```python
from build123d import *

# Parameters (mm, degrees)
SKETCH1_W                                           = 45
SKETCH1_H                                           = 40
BOSS_EXTRUDE1_DEPTH                                 = 29
SKETCH33_W                                          = 34
SKETCH33_H                                          = 35
CUT_EXTRUDE7_DEPTH                                  = 67.828137786
SKETCH39_W                                          = 45
SKETCH39_H                                          = 9
BOSS_EXTRUDE2_DEPTH                                 = 3
CUT_EXTRUDE6_DEPTH                                  = 69.6658576
CUT_EXTRUDE6_DEPTH_BACK                             = 69.6658576
SKETCH21_R                                          = 1.75
SKETCH34_R                                          = 3
CUT_EXTRUDE8_DEPTH                                  = 23
CBORE_FOR_M3_HEX_SOCKET_HEAD_CAP_SCREW1_D           = 3.4
CBORE_FOR_M3_HEX_SOCKET_HEAD_CAP_SCREW1_CBORE_D     = 6.5
CBORE_FOR_M3_HEX_SOCKET_HEAD_CAP_SCREW1_CBORE_DEPTH = 3.4
CBORE_FOR_M3_HEX_SOCKET_HEAD_CAP_SCREW2_D           = 3.4
CBORE_FOR_M3_HEX_SOCKET_HEAD_CAP_SCREW2_CBORE_D     = 6.5
CBORE_FOR_M3_HEX_SOCKET_HEAD_CAP_SCREW2_CBORE_DEPTH = 3.4
FILLET1_R                                           = 4.5
SKETCH40_W                                          = 43
SKETCH40_H                                          = 2
CUT_EXTRUDE9_DEPTH                                  = 69.665857708


with BuildPart() as part:
    # Sketch1 → Boss-Extrude1 (new body)
    with BuildSketch(Plane(origin=(0, 0, 0), x_dir=(1, 0, 0), z_dir=(0, 1, 0))):
        with Locations((22.5, 20)):
            Rectangle(SKETCH1_W, SKETCH1_H)
    extrude(amount=BOSS_EXTRUDE1_DEPTH)

    # Sketch33 → Cut-Extrude7 (cut, through all)
    with BuildSketch(Plane(origin=(0, 29, 0), x_dir=(1, 0, 0), z_dir=(0, 1, 0))):
        with Locations((28, 17.5)):
            Rectangle(SKETCH33_W, SKETCH33_H)
    extrude(amount=-CUT_EXTRUDE7_DEPTH, mode=Mode.SUBTRACT)

    # Sketch39 → Boss-Extrude2 (add)
    with BuildSketch(Plane(origin=(0, 0, -40), x_dir=(-1, 0, 0), z_dir=(0, 0, -1))):
        with Locations((-22.5, 4.5)):
            Rectangle(SKETCH39_W, SKETCH39_H)
    extrude(amount=BOSS_EXTRUDE2_DEPTH)

    # Sketch21 → Cut-Extrude6 (cut, two sides: drawn at the far end of the back side and taken through both)
    with BuildSketch(Plane(origin=(0, 29, 0), x_dir=(1, 0, 0), z_dir=(0, 1, 0)).offset(-CUT_EXTRUDE6_DEPTH_BACK)):
        with Locations(Location((6.5, 39.5, 0), (0, 0, 270))):
            Circle(SKETCH21_R)
        with Locations(Location((6.5, 8.5, 0), (0, 0, 270))):
            Circle(SKETCH21_R)
        with Locations(Location((37.5, 39.5, 0), (0, 0, 270))):
            Circle(SKETCH21_R)
    extrude(amount=CUT_EXTRUDE6_DEPTH + CUT_EXTRUDE6_DEPTH_BACK, mode=Mode.SUBTRACT)

    # Sketch34 → Cut-Extrude8 (cut)
    with BuildSketch(Plane(origin=(0, 29, 0), x_dir=(1, 0, 0), z_dir=(0, 1, 0))):
        with Locations(Location((6.5, 8.5, 0), (0, 0, 270))):
            Circle(SKETCH34_R)
        with Locations(Location((6.5, 39.5, 0), (0, 0, 270))):
            Circle(SKETCH34_R)
        with Locations(Location((37.5, 39.5, 0), (0, 0, 270))):
            Circle(SKETCH34_R)
    extrude(amount=-CUT_EXTRUDE8_DEPTH, mode=Mode.SUBTRACT)

    # CBORE for M3 Hex Socket Head Cap Screw1 (through all)
    with Locations(Plane(origin=(11, 0, 0), x_dir=(0, 0, -1), z_dir=(1, 0, 0))):
        with Locations((16, 19), (30, 19)):
            CounterBoreHole(CBORE_FOR_M3_HEX_SOCKET_HEAD_CAP_SCREW1_D / 2, CBORE_FOR_M3_HEX_SOCKET_HEAD_CAP_SCREW1_CBORE_D / 2, CBORE_FOR_M3_HEX_SOCKET_HEAD_CAP_SCREW1_CBORE_DEPTH)

    # CBORE for M3 Hex Socket Head Cap Screw2 (through all)
    with Locations(Plane.XY.offset(-35)):
        with Locations((16, 19), (30, 19)):
            CounterBoreHole(CBORE_FOR_M3_HEX_SOCKET_HEAD_CAP_SCREW2_D / 2, CBORE_FOR_M3_HEX_SOCKET_HEAD_CAP_SCREW2_CBORE_D / 2, CBORE_FOR_M3_HEX_SOCKET_HEAD_CAP_SCREW2_CBORE_DEPTH)

    # Fillet1
    # the kernel refuses this fillet: 4.5 mm, written as the material it takes off along each edge
    with BuildSketch(Plane(origin=(45, 29, -35), x_dir=(0, 0, -1), z_dir=(0, -1, 0))) as fillet1_piece_1:
        with BuildLine():
            CenterArc((FILLET1_R, -FILLET1_R), FILLET1_R, 90, 90)
            Line((0, -FILLET1_R), (-FILLET1_R * 0.02, -FILLET1_R))
            Line((-FILLET1_R * 0.02, -FILLET1_R), (-FILLET1_R * 0.02, FILLET1_R * 0.02))
            Line((-FILLET1_R * 0.02, FILLET1_R * 0.02), (FILLET1_R, FILLET1_R * 0.02))
            Line((FILLET1_R, FILLET1_R * 0.02), (FILLET1_R, 0))
        make_face()
    extrude(amount=29, mode=Mode.SUBTRACT)
    with BuildSketch(Plane(origin=(11, 29, 0), x_dir=(-1, 0, 0), z_dir=(0, -1, 0))) as fillet1_piece_2:
        with BuildLine():
            CenterArc((FILLET1_R, FILLET1_R), FILLET1_R, 180, 90)
            Line((0, FILLET1_R), (-FILLET1_R * 0.02, FILLET1_R))
            Line((-FILLET1_R * 0.02, FILLET1_R), (-FILLET1_R * 0.02, -FILLET1_R * 0.02))
            Line((-FILLET1_R * 0.02, -FILLET1_R * 0.02), (FILLET1_R, -FILLET1_R * 0.02))
            Line((FILLET1_R, -FILLET1_R * 0.02), (FILLET1_R, 0))
        make_face()
    extrude(amount=29, mode=Mode.SUBTRACT)
    with BuildSketch(Plane(origin=(11, 29, -35), x_dir=(0, 0, -1), z_dir=(1, 0, 0))) as fillet1_piece_3:
        with BuildLine():
            CenterArc((FILLET1_R, -FILLET1_R), FILLET1_R, 90, 90)
            Line((0, -FILLET1_R), (-FILLET1_R * 0.02, -FILLET1_R))
            Line((-FILLET1_R * 0.02, -FILLET1_R), (-FILLET1_R * 0.02, FILLET1_R * 0.02))
            Line((-FILLET1_R * 0.02, FILLET1_R * 0.02), (FILLET1_R, FILLET1_R * 0.02))
            Line((FILLET1_R, FILLET1_R * 0.02), (FILLET1_R, 0))
        make_face()
    extrude(amount=34, mode=Mode.SUBTRACT)
    with BuildSketch(Plane(origin=(11, 29, 0), x_dir=(0, -1, 0), z_dir=(0, 0, -1))) as fillet1_piece_4:
        with BuildLine():
            CenterArc((FILLET1_R, FILLET1_R), FILLET1_R, 180, 90)
            Line((0, FILLET1_R), (-FILLET1_R * 0.02, FILLET1_R))
            Line((-FILLET1_R * 0.02, FILLET1_R), (-FILLET1_R * 0.02, -FILLET1_R * 0.02))
            Line((-FILLET1_R * 0.02, -FILLET1_R * 0.02), (FILLET1_R, -FILLET1_R * 0.02))
            Line((FILLET1_R, -FILLET1_R * 0.02), (FILLET1_R, 0))
        make_face()
    extrude(amount=35, mode=Mode.SUBTRACT)
    with BuildSketch(Plane(origin=(11, 29, -35), x_dir=(0, 0, -1), z_dir=(1, 0, 0))) as fillet1_piece_5a_section:
        with BuildLine():
            CenterArc((FILLET1_R, -FILLET1_R), FILLET1_R, 90, 90)
            Line((0, -FILLET1_R), (-FILLET1_R * 0.02, -FILLET1_R))
            Line((-FILLET1_R * 0.02, -FILLET1_R), (-FILLET1_R * 0.02, FILLET1_R * 0.02))
            Line((-FILLET1_R * 0.02, FILLET1_R * 0.02), (FILLET1_R, FILLET1_R * 0.02))
            Line((FILLET1_R, FILLET1_R * 0.02), (FILLET1_R, 0))
        make_face()
    fillet1_piece_5a = extrude(amount=45.25, mode=Mode.PRIVATE)
    fillet1_piece_5a = split(fillet1_piece_5a, bisect_by=Plane(origin=(45, 27.981221986, -36.018778014), z_dir=(1, 0, 0)), keep=Keep.TOP, mode=Mode.PRIVATE)
    with BuildSketch(Plane(origin=(45, 40.25, -35), x_dir=(0, 0, -1), z_dir=(0, -1, 0))) as fillet1_piece_5b_section:
        with BuildLine():
            CenterArc((FILLET1_R, -FILLET1_R), FILLET1_R, 90, 90)
            Line((0, -FILLET1_R), (-FILLET1_R * 0.02, -FILLET1_R))
            Line((-FILLET1_R * 0.02, -FILLET1_R), (-FILLET1_R * 0.02, FILLET1_R * 0.02))
            Line((-FILLET1_R * 0.02, FILLET1_R * 0.02), (FILLET1_R, FILLET1_R * 0.02))
            Line((FILLET1_R, FILLET1_R * 0.02), (FILLET1_R, 0))
        make_face()
    fillet1_piece_5b = extrude(amount=40.25, mode=Mode.PRIVATE)
    fillet1_piece_5b = split(fillet1_piece_5b, bisect_by=Plane(origin=(43.981221986, 29, -36.018778014), z_dir=(0, 1, 0)), keep=Keep.TOP, mode=Mode.PRIVATE)
    fillet1_piece_5 = fillet1_piece_5a & fillet1_piece_5b
    add(fillet1_piece_5, mode=Mode.SUBTRACT)
    with BuildSketch(Plane(origin=(11, 40.25, 0), x_dir=(-1, 0, 0), z_dir=(0, -1, 0))) as fillet1_piece_6a_section:
        with BuildLine():
            CenterArc((FILLET1_R, FILLET1_R), FILLET1_R, 180, 90)
            Line((0, FILLET1_R), (-FILLET1_R * 0.02, FILLET1_R))
            Line((-FILLET1_R * 0.02, FILLET1_R), (-FILLET1_R * 0.02, -FILLET1_R * 0.02))
            Line((-FILLET1_R * 0.02, -FILLET1_R * 0.02), (FILLET1_R, -FILLET1_R * 0.02))
            Line((FILLET1_R, -FILLET1_R * 0.02), (FILLET1_R, 0))
        make_face()
    fillet1_piece_6a = extrude(amount=40.25, mode=Mode.PRIVATE)
    fillet1_piece_6a = split(fillet1_piece_6a, bisect_by=Plane(origin=(9.981221986, 29, -1.018778014), z_dir=(0, 1, 0)), keep=Keep.TOP, mode=Mode.PRIVATE)
    with BuildSketch(Plane(origin=(11, 29, 11.25), x_dir=(0, -1, 0), z_dir=(0, 0, -1))) as fillet1_piece_6b_section:
        with BuildLine():
            CenterArc((FILLET1_R, FILLET1_R), FILLET1_R, 180, 90)
            Line((0, FILLET1_R), (-FILLET1_R * 0.02, FILLET1_R))
            Line((-FILLET1_R * 0.02, FILLET1_R), (-FILLET1_R * 0.02, -FILLET1_R * 0.02))
            Line((-FILLET1_R * 0.02, -FILLET1_R * 0.02), (FILLET1_R, -FILLET1_R * 0.02))
            Line((FILLET1_R, -FILLET1_R * 0.02), (FILLET1_R, 0))
        make_face()
    fillet1_piece_6b = extrude(amount=46.25, mode=Mode.PRIVATE)
    fillet1_piece_6b = split(fillet1_piece_6b, bisect_by=Plane(origin=(9.981221986, 27.981221986, 0), z_dir=(0, 0, 1)), keep=Keep.TOP, mode=Mode.PRIVATE)
    fillet1_piece_6 = fillet1_piece_6a & fillet1_piece_6b
    add(fillet1_piece_6, mode=Mode.SUBTRACT)
    with BuildSketch(Plane(origin=(11, 29, 0), x_dir=(0, -1, 0), z_dir=(0, 0, -1))) as fillet1_piece_7a_section:
        with BuildLine():
            CenterArc((FILLET1_R, FILLET1_R), FILLET1_R, 180, 90)
            Line((0, FILLET1_R), (-FILLET1_R * 0.02, FILLET1_R))
            Line((-FILLET1_R * 0.02, FILLET1_R), (-FILLET1_R * 0.02, -FILLET1_R * 0.02))
            Line((-FILLET1_R * 0.02, -FILLET1_R * 0.02), (FILLET1_R, -FILLET1_R * 0.02))
            Line((FILLET1_R, -FILLET1_R * 0.02), (FILLET1_R, 0))
        make_face()
    fillet1_piece_7a = extrude(amount=46.25, mode=Mode.PRIVATE)
    fillet1_piece_7a = split(fillet1_piece_7a, bisect_by=Plane(origin=(9.981221986, 27.981221986, -35), z_dir=(0, 0, -1)), keep=Keep.TOP, mode=Mode.PRIVATE)
    with BuildSketch(Plane(origin=(-0.25, 29, -35), x_dir=(0, 0, -1), z_dir=(1, 0, 0))) as fillet1_piece_7b_section:
        with BuildLine():
            CenterArc((FILLET1_R, -FILLET1_R), FILLET1_R, 90, 90)
            Line((0, -FILLET1_R), (-FILLET1_R * 0.02, -FILLET1_R))
            Line((-FILLET1_R * 0.02, -FILLET1_R), (-FILLET1_R * 0.02, FILLET1_R * 0.02))
            Line((-FILLET1_R * 0.02, FILLET1_R * 0.02), (FILLET1_R, FILLET1_R * 0.02))
            Line((FILLET1_R, FILLET1_R * 0.02), (FILLET1_R, 0))
        make_face()
    fillet1_piece_7b = extrude(amount=45.25, mode=Mode.PRIVATE)
    fillet1_piece_7b = split(fillet1_piece_7b, bisect_by=Plane(origin=(11, 27.981221986, -36.018778014), z_dir=(-1, 0, 0)), keep=Keep.TOP, mode=Mode.PRIVATE)
    fillet1_piece_7 = fillet1_piece_7a & fillet1_piece_7b
    add(fillet1_piece_7, mode=Mode.SUBTRACT)

    # Sketch40 → Cut-Extrude9 (cut, through all)
    with BuildSketch(Plane.ZY):
        with Locations((-21.5, 1)):
            Rectangle(SKETCH40_W, SKETCH40_H)
    extrude(amount=-CUT_EXTRUDE9_DEPTH, mode=Mode.SUBTRACT)


solid = part.part
```
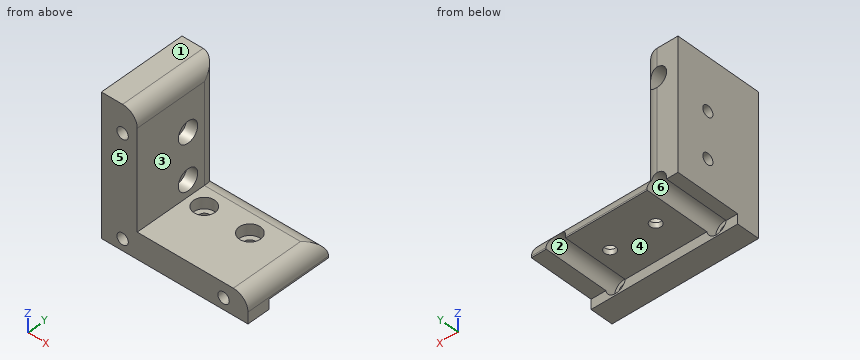
The listing builds one solid part. Answer for the finished solid, in the listing's coordinates (mm). Face numbers are marked on the shaded views. A direction names the side the tool comes from. Round coordinates to 2 decimals unless told otherwise and drop trailing zeros. Order: outer loops, then holes, each group sorted by start corner. A loop starts at its lowest first (then second) coordinate and runs counter-clockwise, first axis right, second up. Notation, with made-up numbers: (4, 65.25) -> (8, 65.25) arc R17 cw to (8, 88.25) -> close; hole circle Ø4 at (-7, 31). An arc over 180 degrees is marked (long way). Answer as CSV lines item,"result". Start each with the question number.
(1) The part is cut by section B-B (y = 5.25). Determine the outline of the cut face in (x, z).
(2) The part is cut by section C-C (z = -30). Determine the outline of the cut face in (x, y).
(3) Find the intervals of material crossed by probe 1 along X at (y, z) = (24.25, -39.5); probe 2 along Y at (x, z) = (3, -16); probe 3 along Z at (x, y) = (6.5, 3.35), in increasing order. Write a range as from..to.
(4) A tool of negligible diameter and unlimited length cuts with its end or side. For the marked faces 1, 2 and 3, from which of +Z, -Z, +X, -X, +Y, -Y can it reach the whole face along a straight path? Write none if from no direction.
(5) For a pull along Z with two mould halves and no side action, classify the marked faces 4, 5 and 6 as +Z half, -Z half, draft (parallel to the pull), parting line (faces both ways), or undercut.
(6) The part is cut by section D-D (y = 19). Count the separate pieces of the cut face and the enclosed holes in it, then the cut area to 3 significant figures.
(7) Flat-ended cylindrical pins translate along their axes: pin 1 Ø10.5 at (y, z) = (19, -16) entering from +X; pin 2 Ø1 at (x, y) = (27.5, 9.5) entering from +Z; pin 3 Ø7 at (x, z) = (6.5, -39.5) entering from +Y; pin 4 Ø5.5 at (x, y) = (16, 19) entering from -Z. Find the tip coordinate at first contact, or state that the pin passes through.
(8) The part is cut by section A-A (x = 30). Determine the outline of the cut face in (y, z).
Evaluation:
1,outline,"(0, -43) -> (45, -43) -> (45, -39.5) arc R4.5 ccw to (40.5, -35) -> (11, -35) -> (11, -4.5) arc R4.5 ccw to (6.5, 0) -> (0, 0) -> close; hole circle Ø3.5 at (6.5, -39.5); hole circle Ø3.5 at (6.5, -8.5); hole circle Ø3.5 at (37.5, -39.5)"
2,outline,"(0, 2) -> (11, 2) -> (11, 15.75) -> (7.6, 15.75) -> (7.6, 17.3) -> (0, 17.3) -> close; (0, 20.7) -> (7.6, 20.7) -> (7.6, 22.25) -> (11, 22.25) -> (11, 24.5) arc R4.5 ccw to (6.5, 29) -> (0, 29) -> close"
3,probe 1,"0..3.5, 9.5..34.5, 40.5..45"
3,probe 2,"2..17.3, 20.7..29"
3,probe 3,"-43..-41.25, -37.75..-10.25, -6.75..0"
4,face 1,"+Z, +X, -X, +Y, -Y"
4,face 2,"+Y"
4,face 3,"+Z, +X, +Y, -Y"
5,face 4,"-Z half"
5,face 5,"draft"
5,face 6,"undercut"
6,separate pieces,"5"
6,enclosed holes,"1"
6,area,"388 mm²"
7,pin 1,"x = 11"
7,pin 2,"z = -35"
7,pin 3,"y = 29"
7,pin 4,"z = -40"
8,outline,"(2, -43) -> (9, -43) -> (9, -40) -> (17.3, -40) -> (17.3, -38.4) -> (15.75, -38.4) -> (15.75, -35) -> (2, -35) -> close; (20.7, -40) -> (29, -40) -> (29, -39.5) arc R4.5 ccw to (24.5, -35) -> (22.25, -35) -> (22.25, -38.4) -> (20.7, -38.4) -> close"
